Work out the finished part from the listing and answer in its coordinate system (mm). A direction names the side the tool comes from. Round coordinates to 2 decimals unless told otherwise and drop trailing zeros. Loops run counter-clockwise (first coordinate to the right, second up) from the corner with the lowest first, then second, coordinate; pieces in that order, holes last. Notation, with made-up numbers: M -3,4 L 46,4 A24 ccw 46,30 Z; hole C 36.25,65.25 d7. An arc over 180 degrees is marked long. One line per item, written item: value.
```python
from build123d import *

# Parameters (mm, degrees)
BOSS_EXTRUDE1_DEPTH      = 133
BOSS_EXTRUDE1_DEPTH_BACK = 133
SKETCH1_W                = 25.4
SKETCH1_H                = 24
CUT_EXTRUDE1_DEPTH       = 150
CUT_EXTRUDE1_DEPTH_BACK  = 150
SKETCH2_W                = 26
SKETCH2_H                = 22.28
CUT_EXTRUDE2_DEPTH       = 150
CUT_EXTRUDE2_DEPTH_BACK  = 150
SKETCH3_R                = 2.4


with BuildPart() as part:
    # Sketch1 → Boss-Extrude1 (new, two sides: drawn at the far end of the back side and taken through both)
    with BuildSketch(Plane(origin=(0, 0, 0), x_dir=(1, 0, 0), z_dir=(0, 1, 0)).offset(-BOSS_EXTRUDE1_DEPTH_BACK)):
        Rectangle(SKETCH1_W, SKETCH1_H)
    extrude(amount=BOSS_EXTRUDE1_DEPTH + BOSS_EXTRUDE1_DEPTH_BACK)

    # Sketch2 → Cut-Extrude1 (cut, two sides: drawn at the far end of the back side and taken through both)
    with BuildSketch(Plane(origin=(0, 0, 0), x_dir=(1, 0, 0), z_dir=(0, 1, 0)).offset(-CUT_EXTRUDE1_DEPTH_BACK)):
        with Locations((-1.16, 0)):
            Rectangle(SKETCH2_W, SKETCH2_H)
    extrude(amount=CUT_EXTRUDE1_DEPTH + CUT_EXTRUDE1_DEPTH_BACK, mode=Mode.SUBTRACT)

    # Sketch3 → Cut-Extrude2 (cut, two sides: drawn at the far end of the back side and taken through both)
    with BuildSketch(Plane.XY.offset(-CUT_EXTRUDE2_DEPTH_BACK)):
        with Locations(Location((0, 124.125, 0), (0, 0, 180))):
            Circle(SKETCH3_R)
        with Locations(Location((0, 94.125, 0), (0, 0, 180))):
            Circle(SKETCH3_R)
        with Locations(Location((0, -124.125, 0), (0, 0, 180))):
            Circle(SKETCH3_R)
        with Locations(Location((0, -94.125, 0), (0, 0, 180))):
            Circle(SKETCH3_R)
    extrude(amount=CUT_EXTRUDE2_DEPTH + CUT_EXTRUDE2_DEPTH_BACK, mode=Mode.SUBTRACT)


solid = part.part
```
1) For faces 5 (the face through (-1, -2, -11.14)), 6 (the face through (0, -2, -12)), determine the directions among +Z, -Z, +X, -X, +Y, -Y from which every point of the face is accessible in a straight line to the end or side of a thin tool.
Check values:
face 5: -X, +Y, -Y
face 6: -Z, +X, -X, +Y, -Y
2) Each of these flat-tipped pins is pushed along its axis until it touches: pin 1 (10 mm diameter, centred on y = -7, z = -6.5, fed in from -X); pin 2 (4.5 mm diameter, centred on x = 0, y = -124.125, fed in from -Z); pin 3 (10 mm diameter, centred on y = 102.5, z = 2.5, fed in from -X). Where does it stop, or does it pass through?
Check values:
pin 1: x = -12.7
pin 2: through
pin 3: x = 11.84
3) Find section A-A (x = 8). Give the vertices of the cut face in (y, z), then the cut area to 3 significant figures.
Check values:
outline: M -133,-12 L 133,-12 L 133,-11.14 L -133,-11.14 Z; M -133,11.14 L 133,11.14 L 133,12 L -133,12 Z
area: 458 mm2
4) The mould has two halves that part along Z. Classify faces 1 (the face through (0, -2, 12)), 2 (the face through (-1, -2, 11.14)), 3 (the face through (11.84, -2, 0)), 4 (the face through (0.312, 91.745, 11.564)): +Z half, -Z half, draft (parallel to the pull), parting line (faces both ways), or undercut.
Check values:
face 1: +Z half
face 2: undercut
face 3: undercut
face 4: draft
5) Find section C-C (z = 3). Give the vertices of the cut face in (x, y), then the cut area to 3 significant figures.
Check values:
outline: M 11.84,-133 L 12.7,-133 L 12.7,133 L 11.84,133 Z
area: 229 mm2
6) Find the intervals of material crossed by probe 1 along Y at (x, z) = (0, -11.5) (3 decimals); probe 2 along Z at (x, y) = (9.5, -56); probe 3 along X at (y, z) = (44, 0.25), in increasing order. Write a range as from..to.
Check values:
probe 1: -133..-126.525, -121.725..-96.525, -91.725..91.725, 96.525..121.725, 126.525..133
probe 2: -12..-11.14, 11.14..12
probe 3: 11.84..12.7
7) Find section B-B (y = -23.5). Give the vertices of the cut face in (x, z), then the cut area to 3 significant figures.
Check values:
outline: M -12.7,-12 L 12.7,-12 L 12.7,12 L -12.7,12 L -12.7,11.14 L 11.84,11.14 L 11.84,-11.14 L -12.7,-11.14 Z
area: 62.8 mm2
